Model file for the job. Use its own axes, mm. Face numbers are marked on the shaded views. A direction names the side the tool comes from. Give positions to 0.01 mm unless a question says otherwise; leave off trailing zeros. Order: outer loops, then holes, each group sorted by start corner. A loop starts at its lowest first (then second) coordinate and runs counter-clockwise, first axis right, second up. Notation, with made-up numbers: (70, -14.75) -> (117, -14.75) arc R11 ccw to (117, -4.75) -> close; hole circle Ø9 at (-21.75, 58). An arc over 180 degrees is marked (long way). Use CSV: the item, a comma, the result in double quotes. Start each with the question number.
1. Drop flat-ended pins along their axis: pin 1 (7 mm diameter, centred on x = -11.31, y = -11.31, fed in from -Z); pin 2 (9 mm diameter, centred on x = 0, y = -36, fed in from +Z); pin 3 (25 mm diameter, centred on x = 11.5, y = -19.5, fed in from +Z); pin 4 (2 mm diameter, centred on x = 11, z = 9.5, fed in from +Y). Give the stop position or say it passes through.
2. Cut at A-A on y = -36. List the corners of the cut face in (x, z), then the cut area to 3 significant figures.
3. Cut at C-C on y = 0. List the corners of the cut face in (x, z).
4. Wall check: line 1 (X direction, y = 15, z = 1.15); line 2 (Y direction, x = 0, z = 1.1); line 3 (Y direction, x = -14, z = 7). Give the ranges that are in metal, low to high. Write a range as from..to.
5. Cut at D-D on z = 8.5. List the corners of the cut face in (x, y).
6. 3-axis set-ups, long thin cutter, end or side, ignore diameter. For the marked faces 1 and 2: which of +Z, -Z, +X, -X, +Y, -Y reach the whole face in a straight line?
7. Cut at B-B on x = 0. List the corners of the cut face in (y, z).
Autodesk Inventor part; units mm, degrees
ref_plane "YZ Plane" through (0, 0, 0) normal (1, 0, 0) x (0, 1, 0)
ref_plane "XZ Plane" through (0, 0, 0) normal (0, 1, 0) x (-1, 0, 0)
ref_plane "XY Plane" through (0, 0, 0) normal (0, 0, 1) x (1, 0, 0)
sketch "スケッチ1" plane through (0, 0, 0) normal (0, 0, 1) x (1, 0, 0)
  line L0 (-25, -72.3) -> (25, -72.3)
  line L1 (25, -72.3) -> (25, 25)
  line L2 (25, 25) -> (-25, 25)
  line L3 (-25, 25) -> (-25, -72.3)
  line L4 (-25, -72.3) -> (25, 25) construction
  line L5 (25, -72.3) -> (-25, 25) construction
  circle A0 centre (0, 0) radius 19 construction
  point P0 (0, -23.65)
  point P1 (0, -23.65)
  dimension "d0" = 38
  dimension "d1" = 50
  dimension "d2" = 25
  dimension "d3" = 72.3
extrude "プレート1" add sketch "スケッチ1" along normal blind 2.3
sketch "スケッチ9" plane through (25, -70, 0) normal (0, -1, 0) x (1, 0, 0)
  line L0 (-50, 0) -> (0, 0)
  line L1 (0, 0) -> (0, 14.6)
  line L2 (0, 14.6) -> (-50, 14.6)
  line L3 (-50, 14.6) -> (-50, 0)
edge flange "フランジ3" height 14.6 angle 90 thickness 2.3 bend radius 2.3 thickness toward (0, -1, 0) relief tear relief width 2.3 relief depth 1.15 edges at (0, -72.3, 2.3) wall of the first edge with corners at (-25, -70, 0) (25, -70, 0) (25, -70, 14.6) (-25, -70, 14.6)
bend "曲げ3"
corner "コーナー3"
fillet "コーナーR1" radius 5 2 edges at (25, -71.15, 14.6) (-25, -71.15, 14.6)
sketch "スケッチ4" plane through (0, 0, 2.3) normal (0, 0, 1) x (1, 0, 0)
  circle A0 centre (0, 0) radius 15
  point P0 (0, 15)
  point P1 (-15, 0)
  point P2 (0, -15)
  point P3 (15, 0)
  dimension "d26" = 30
  dimension "d29" = 360
hole "穴1" at (0, 15, 2.3) at (-15, 0, 2.3) at (0, -15, 2.3) at (15, 0, 2.3) direction (0, 0, -1) diameter 3.2 end through all
sketch "スケッチ5" plane through (0, 0, 2.3) normal (0, 0, 1) x (1, 0, 0)
  circle A0 centre (0, 0) radius 16
  point P0 (-11.3137, 11.3137)
  point P1 (-11.3137, -11.3137)
  point P2 (11.3137, -11.3137)
  point P3 (11.3137, 11.3137)
  dimension "d38" = 32
  dimension "d41" = 360
hole "穴2" at (-11.3137, 11.3137, 2.3) at (-11.3137, -11.3137, 2.3) at (11.3137, -11.3137, 2.3) at (11.3137, 11.3137, 2.3) direction (0, 0, -1) diameter 4.3 end through all
sketch "スケッチ6" plane through (0, 0, 2.3) normal (0, 0, 1) x (1, 0, 0)
  circle A0 centre (0, 0) radius 10
  dimension "d50" = 20
extrude "押し出し1" cut sketch "スケッチ6" against normal blind 10
sketch "スケッチ7" plane through (-25, -70, -2.3) normal (0, 1, 0) x (1, 0, 0)
  line L0 (5, -16.9) -> (45, -16.9)
  line L1 (0, -6.9) -> (0, -11.9)
  line L2 (50, -6.9) -> (50, -11.9)
  point P0 (18, -2.3)
  point P1 (45, -11.9)
  point P2 (5, -11.9)
  dimension "d76" = 5
  dimension "d77" = 5
  dimension "d78" = 5
hole "穴3" at (20, -70, 9.6) at (-20, -70, 9.6) direction (0, -1, 0) diameter 4.3 end through all
fillet "コーナーR3" radius 10 2 edges at (-25, 25, 1.15) (25, 25, 1.15)
sketch "スケッチ10" plane through (0, 0, 0) normal (0, 0, -1) x (-1, 0, 0)
  line L0 (-25, -67.7) -> (-25, 15)
  line L1 (25, 15) -> (25, -67.7)
  circle A0 centre (-20, -45) radius 4
  circle A1 centre (0, 0) radius 45
  point P0 (20, -45)
  dimension "d80" = 5
  dimension "d81" = 5
  dimension "d82" = 45
  dimension "d83" = 8
  dimension "d84" = 90
hole "穴4" at (20, -45, 0) at (-20, -45, 0) direction (0, 0, 1) diameter 4.3 end through all
sketch "スケッチ11" plane through (0, 0, 2.3) normal (0, 0, 1) x (1, 0, 0)
  circle A0 centre (0, -36) radius 5
  point P0 (0, 0)
  dimension "d92" = 10
  dimension "d93" = 36
extrude "押し出し3" cut sketch "スケッチ11" against normal blind 10
equation "\"d36\" = Thickness"
equation "\"d48\" = Thickness"
equation "\"d61\" = Thickness"
equation "\"d90\" = Thickness"
equation "\"d4\" = Thickness"
equation "\"d66\" = BendReliefWidth"
equation "\"d67\" = BendReliefDepth"
equation "\"d68\" = MinimumRemnant"
equation "\"d69\" = TransitionRadius"
equation "\"d72\" = BendRadius"
equation "\"d73\" = CornerReliefSize"
equation "\"d74\" = GapSize"
equation "\"d75\" = JacobiRadiusSize"
equation "\"BendRadius\" = Thickness"
equation "\"BendReliefWidth\" = Thickness"
equation "\"BendReliefDepth\" = 0.5 * Thickness"
equation "\"CornerReliefSize\" = 4 * Thickness"
equation "\"MinimumRemnant\" = 2 * Thickness"
equation "\"TransitionRadius\" = BendRadius"
equation "\"JacobiRadiusSize\" = BendRadius"
equation "\"GapSize\" = Thickness"
properties part number "plate8" material "鋼、炭素鋼"
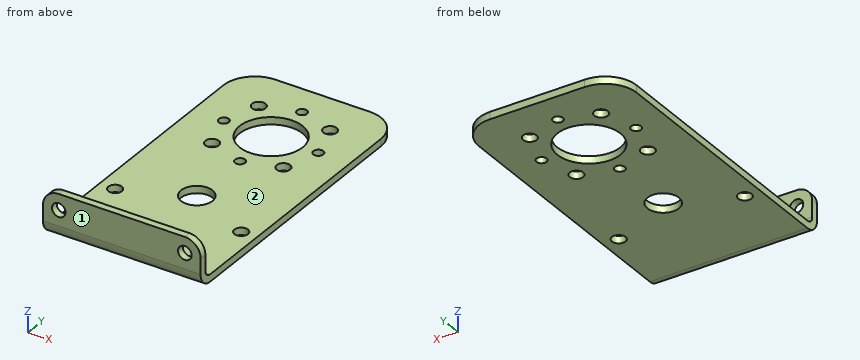
Verdict:
1,pin 1,"z = 0"
1,pin 2,"through"
1,pin 3,"z = 2.3"
1,pin 4,"y = -70"
2,outline,"(-25, 0) -> (-5, 0) -> (-5, 2.3) -> (-25, 2.3) -> close; (5, 0) -> (25, 0) -> (25, 2.3) -> (5, 2.3) -> close"
2,area,"92.0 mm^2"
3,outline,"(-25, 0) -> (-16.6, 0) -> (-16.6, 2.3) -> (-25, 2.3) -> close; (-13.4, 0) -> (-10, 0) -> (-10, 2.3) -> (-13.4, 2.3) -> close; (10, 0) -> (13.4, 0) -> (13.4, 2.3) -> (10, 2.3) -> close; (16.6, 0) -> (25, 0) -> (25, 2.3) -> (16.6, 2.3) -> close"
4,line 1,"-25..-1.6, 1.6..25"
4,line 2,"-70.68..-41, -31..-16.6, -13.4..-10, 10..13.4, 16.6..25"
4,line 3,"-72.3..-70"
5,outline,"(-25, -72.3) -> (-21.85, -72.3) -> (-21.85, -70) -> (-25, -70) -> close; (-18.15, -72.3) -> (18.15, -72.3) -> (18.15, -70) -> (-18.15, -70) -> close; (21.85, -72.3) -> (25, -72.3) -> (25, -70) -> (21.85, -70) -> close"
6,face 1,"+Z, -Z, +X, -X, -Y"
6,face 2,"+Z, +X, -X, +Y"
7,outline,"(-72.3, 4.6) arc R4.6 ccw to (-67.7, 0) -> (-41, 0) -> (-41, 2.3) -> (-67.7, 2.3) arc R2.3 cw to (-70, 4.6) -> (-70, 14.6) -> (-72.3, 14.6) -> close; (-31, 0) -> (-16.6, 0) -> (-16.6, 2.3) -> (-31, 2.3) -> close; (-13.4, 0) -> (-10, 0) -> (-10, 2.3) -> (-13.4, 2.3) -> close; (10, 0) -> (13.4, 0) -> (13.4, 2.3) -> (10, 2.3) -> close; (16.6, 0) -> (25, 0) -> (25, 2.3) -> (16.6, 2.3) -> close"
